```python
from build123d import *

# Parameters (mm, degrees)
F0_W     = 50.8
F0_H     = 203.2
F1_DEPTH = 9.525
F2_SIZE2 = 3.6661742094
F2_SIZE  = 6.35


# Not quite as in the source:
# - a length typed as a fraction of an inch, garbled in the dataset ("3 / 203.2 mm" for 3/8 in), is restored


with BuildPart() as f1:
    # F0 (on Front) → F1 (new body)
    with BuildSketch(Plane.XZ):
        with Locations((-1.7615184188, 42.1527517154)):
            Rectangle(F0_W, F0_H)
    extrude(amount=F1_DEPTH)

    # F2
    f2_edges = [f1.edges().sort_by_distance(p)[0] for p in [
        (23.638482, -9.525, 42.152752),
    ]]
    f2_side = f1.faces().sort_by_distance((23.638482, -4.7625, 42.152752))[0]
    chamfer(f2_edges, length=F2_SIZE, length2=F2_SIZE2, reference=f2_side)


solid = f1.part
```
Check sheet for the modelled part. Datum: model origin and axes. Units: mm. Round coordinates to 2 decimals unless told otherwise and drop trailing zeros. Loops run counter-clockwise (first coordinate to the right, second up) from the corner with the lowest first, then second, coordinate; pieces in that order, holes last. Notation, with made-up numbers: M 55.25,-38 L 88.25,-38 A9 ccw 88.25,-22 Z; hole C 8,13 d1. An arc over 180 degrees is marked long. Answer as a JSON object with one key per item and string values.
1. Section check B-B (y = -5.25). Record the boundary of the cut face in (x, z).
Reply:
{"outline": "M -27.16,-59.45 L 22.44,-59.45 L 22.44,143.75 L -27.16,143.75 Z"}
2. Scan lines: line 1 (X direction, y = -5.5, z = 70.5); line 2 (X direction, y = -7.25, z = 36); line 3 (Y direction, x = 21.5, z = 25). Record each from-to range of solid material in increasing order.
Reply:
{"line 1": "x = -27.16 to 22.3", "line 2": "x = -27.16 to 21.29", "line 3": "y = -6.88 to 0"}
3. Gauge pin test, flat ends, axial feed: P1, Ø12, axis at x = -17, z = 110.5, coming from the +Y side; P2, Ø1, axis at y = -5, z = 6.5, coming from the +X side. Record the tip position at first contact, or that the pin passes through.
Reply:
{"P1": "stops at y = 0", "P2": "stops at x = 22.87"}
4. Section check A-A (z = 47). Record the boundary of the cut face in (x, y) (3 decimals), plus the area to 3 significant figures.
Reply:
{"outline": "M -27.162,-9.525 L 19.972,-9.525 L 23.638,-3.175 L 23.638,0 L -27.162,0 Z", "area": "472 mm²"}
